Input: part model. Units: mm. Frame: model coordinates. Face numbers are marked on the shaded views. A direction names the side the tool comes from. Round coordinates to 2 decimals unless told otherwise and drop trailing zeros. Order: outer loops, then holes, each group sorted by start corner. A loop starts at its lowest first (then second) coordinate and runs counter-clockwise, first axis right, second up. Notation, with made-up numbers: M 8,71.5 L 22,71.5 A20 cw 22,94.5 Z; hole C 83.25,-2 d3. An arc over 180 degrees is marked long. One line per question, with ' | ' between items.
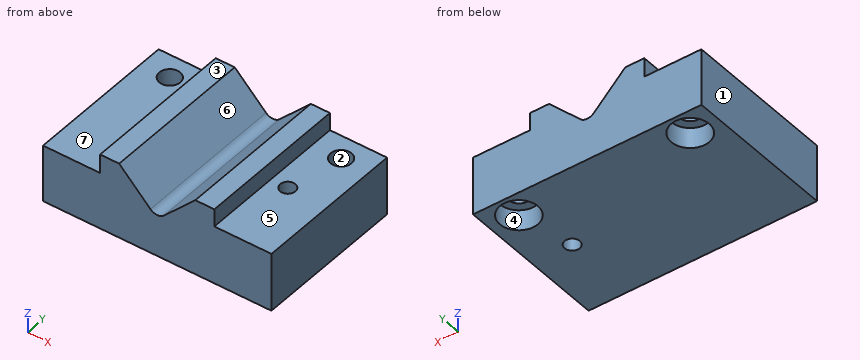
```python
from build123d import *

# Parameters (mm, degrees)
F1_DEPTH       = 40
F3_D           = 5.5
F3_CBORE_D     = 10
F3_CBORE_DEPTH = 5.4
F5_D           = 4


with BuildPart() as f1:
    # F0 (on Front) → F1 (new body)
    with BuildSketch(Plane.XZ):
        with BuildLine():
            Line((-15, 5), (-30, 5))
            Line((-30, 5), (-30, -10))
            Line((-30, -10), (30, -10))
            Line((30, -10), (30, 5.364162))
            Line((30, 5.364162), (15, 5.364162))
            Line((15, 5.364162), (15, 10))
            Line((15, 10), (10, 10))
            Line((10, 10), (1.767767, 1.767767))
            ThreePointArc((1.767767, 1.767767), (0, 1.035534), (-1.767767, 1.767767))
            Line((-1.767767, 1.767767), (-10, 10))
            Line((-10, 10), (-15, 10))
            Line((-15, 10), (-15, 5))
        make_face()
    extrude(amount=F1_DEPTH)

    # F3 (through all)
    with Locations(Plane(origin=(0, 0, -10), x_dir=(1, 0, 0), z_dir=(0, 0, -1))):
        with Locations((-22.5, 6), (22.5, 6)):
            CounterBoreHole(F3_D / 2, F3_CBORE_D / 2, F3_CBORE_DEPTH)

    # F5 (through all)
    with Locations(Plane(origin=(0, 0, -10), x_dir=(1, 0, 0), z_dir=(0, 0, -1))):
        with Locations((19.5, 20.5)):
            Hole(F5_D / 2)


solid = f1.part
```
Item 1: Section query D-D, the plane z = -8.25. Return loops of the section in (x, y).
Report:
outline: M -30,-40 L 30,-40 L 30,0 L -30,0 Z; hole C -22.5,-6 d10; hole C 19.5,-20.5 d4; hole C 22.5,-6 d10
Item 2: Access query for the marked faces 4, 5, 6 and 7. Directions: +Z, -Z, +X, -X, +Y, -Y. A direction counts if a zero-diameter tool reaches every point of the face in a straight line with its end or side. Return the directions, or none.
Report:
face 4: -Z | face 5: +Z, +X, +Y, -Y | face 6: +Z, +Y, -Y | face 7: +Z, -X, +Y, -Y
Item 3: First-contact query: pin 1 (7 mm diameter, centred on x = 22.5, y = -6, fed in from -Z); pin 2 (6 mm diameter, centred on x = 22.5, y = -6, fed in from +Z); pin 3 (6 mm diameter, centred on x = -22.5, y = -6, fed in from +Z). Flat tips, straight axial feed; report the tip coordinate or a pass-through.
Report:
pin 1: z = -4.6 | pin 2: z = 5.36 | pin 3: z = 5
Item 4: Mould query, pull axis X, two halves, no side actions, for the marked faces 1, 2 and 3. Classes: +X half, -X half, draft (parallel to the pull), parting line (faces both ways), or undercut.
Report:
face 1: -X half | face 2: undercut | face 3: draft
Item 5: Section query B-B, the plane y = -6. Return loops of the section in (x, z), plus the area to 3 significant figures.
Report:
outline: M -30,-10 L -27.5,-10 L -27.5,-4.6 L -25.25,-4.6 L -25.25,5 L -30,5 Z; M -19.75,-4.6 L -17.5,-4.6 L -17.5,-10 L 17.5,-10 L 17.5,-4.6 L 19.75,-4.6 L 19.75,5.36 L 15,5.36 L 15,10 L 10,10 L 1.77,1.77 A2.5 cw -1.77,1.77 L -10,10 L -15,10 L -15,5 L -19.75,5 Z; M 25.25,-4.6 L 27.5,-4.6 L 27.5,-10 L 30,-10 L 30,5.36 L 25.25,5.36 Z | area: 741 mm²
Item 6: Section query C-C, the plane x = 22.5. Return loops of the section in (y, z).
Report:
outline: M -40,-10 L -11,-10 L -11,-4.6 L -8.75,-4.6 L -8.75,5.36 L -40,5.36 Z; M -3.25,-4.6 L -1,-4.6 L -1,-10 L 0,-10 L 0,5.36 L -3.25,5.36 Z
Item 7: Section query A-A, the plane z = 3.5. Return loops of the section in (x, y), plus the area to 3 significant figures.
Report:
outline: M -30,-40 L -3.5,-40 L -3.5,0 L -30,0 Z; M 3.5,-40 L 30,-40 L 30,0 L 3.5,0 Z; hole C -22.5,-6 d5.5; hole C 19.5,-20.5 d4; hole C 22.5,-6 d5.5 | area: 2,060 mm²
Item 8: Line query: line 1 along X through (y, z) = (-5, -6); line 2 along X through (y, z) = (-20.5, 1.5); line 3 along Y through (x, z) = (22.5, -6.3). Output: solid intervals per line, ascending. Write a range as from..to.
Report:
line 1: -30..-27.4, -17.6..17.6, 27.4..30 | line 2: -30..-1.45, 1.45..17.5, 21.5..30 | line 3: -40..-11, -1..0
